```python
from build123d import *

# Parameters (mm, degrees)
SKETCH_1_W          = 27.8
SKETCH_1_H          = 8
EXTRUDE_1_DEPTH     = 7.8
EXTRUDE_2_DEPTH     = 27.8
SKETCH_4_R          = 1.15
EXTRUDE_3_DEPTH     = 2
CUT_EXTRUDE_4_DEPTH = 24.8
SKETCH_15_W         = 27.8
SKETCH_15_H         = 4.251772847
EXTRUDE_4_DEPTH     = 1.9
FILLET_1_R          = 8
FILLET_2_R          = 6.5
EXTRUDE_5_DEPTH     = 27.8
CUT_EXTRUDE_6_DEPTH = 24.8
SKETCH_19_OUTSIDE_W = 26.556
SKETCH_19_OUTSIDE_H = 34.032
CUT_EXTRUDE_7_DEPTH = 40.8
SKETCH_20_W         = 1.5
SKETCH_20_H         = 5.56
EXTRUDE_6_DEPTH     = 6.2
SKETCH_21_W         = 1.5
SKETCH_21_H         = 3.16
CUT_EXTRUDE_8_DEPTH = 4.68
EXTRUDE_7_DEPTH     = 1
FILLET_3_R          = 0.2


with BuildPart() as part:
    # 草图1 → 凸台-拉伸1 (new body)
    with BuildSketch(Plane.XY):
        with Locations((13.9, -4)):
            Rectangle(SKETCH_1_W, SKETCH_1_H)
    extrude(amount=EXTRUDE_1_DEPTH)

    # 草图2 → 凸台-拉伸2 (add)
    with BuildSketch(Plane.ZY):
        Polygon((5.795554958, -15.947085729), (0, -17.5), (0, -8), (7.8, -8), align=None)
    extrude(amount=-EXTRUDE_2_DEPTH)

    # 草图4 → 凸台-拉伸3 (add)
    with BuildSketch(Plane(origin=(0, 0, -1.9), x_dir=(-1, 0, 0), z_dir=(0, 0, -1))):
        with BuildLine():
            Line((0, -2), (0, -4.7))
            Line((0, -4.7), (6, -4.7))
            ThreePointArc((6, -4.7), (6.353553391, -4.553553391), (6.5, -4.2))
            Line((6.5, -4.2), (6.5, -2))
            Line((6.5, -2), (6.5, 2.4))
            ThreePointArc((6.5, 2.4), (6.353553391, 2.753553391), (6, 2.9))
            Line((6, 2.9), (4, 2.9))
            ThreePointArc((4, 2.9), (2.232233047, 2.167766953), (1.5, 0.4))
            Line((1.5, 0.4), (1.5, -1.8))
            ThreePointArc((1.5, -1.8), (1.441421356, -1.941421356), (1.3, -2))
            Line((1.3, -2), (0, -2))
        make_face()
        with Locations((3.6, 0.5)):
            Circle(SKETCH_4_R, mode=Mode.SUBTRACT)
    extrude_3 = extrude(amount=-EXTRUDE_3_DEPTH)

    # 镜向1: 凸台-拉伸3 across plane
    add(extrude_3.mirror(Plane.ZY.offset(-13.9)))

    # 草图13 → 切除-拉伸4 (cut)
    with BuildSketch(Plane.ZY.offset(-1.5)):
        Polygon((1.5, 0), (1.5, -11.921695309), (0, -12.323619098), (0, -15.947085729), (4.556522218, -14.726169281), (6.3, -7.813748582), (6.3, 0), align=None)
    extrude(amount=-CUT_EXTRUDE_4_DEPTH, mode=Mode.SUBTRACT)

    # 草图15 → 凸台-拉伸4 (add)
    with BuildSketch(Plane(origin=(0, 0, 0), x_dir=(-1, 0, 0), z_dir=(0, 0, -1))):
        with Locations((-13.9, -4.125886424)):
            Rectangle(SKETCH_15_W, SKETCH_15_H)
    extrude(amount=EXTRUDE_4_DEPTH)

    # 圆角1
    fillet_1_edges = [part.edges().sort_by_distance(p)[0] for p in [
        (13.9, -14.726169281, 4.556522218),
    ]]
    fillet(fillet_1_edges, radius=FILLET_1_R)

    # 圆角2
    fillet_2_edges = [part.edges().sort_by_distance(p)[0] for p in [
        (13.9, -15.947085729, 5.795554958),
    ]]
    fillet(fillet_2_edges, radius=FILLET_2_R)

    # 草图17 → 凸台-拉伸5 (add)
    with BuildSketch(Plane(origin=(27.8, 0, 0), x_dir=(0, 0, -1), z_dir=(1, 0, 0))):
        Polygon((0, -17.5), (7, -19.375644347), (7, -12.646349174), (0, -10.770704827), align=None)
    extrude(amount=-EXTRUDE_5_DEPTH)

    # 草图18 → 切除-拉伸6 (cut)
    with BuildSketch(Plane.ZY.offset(-26.3)):
        Polygon((0, -12.323619098), (0, -15.947085729), (-7, -17.822730076), (-7, -14.199263445), align=None)
    extrude(amount=CUT_EXTRUDE_6_DEPTH, mode=Mode.SUBTRACT)

    # 草图19 outside → 切除-拉伸7 (cut)
    with BuildSketch(Plane(origin=(34.3, 0, 0), x_dir=(0, 0, -1), z_dir=(1, 0, 0))):
        with Locations((-0.4, -8.238)):
            Rectangle(SKETCH_19_OUTSIDE_W, SKETCH_19_OUTSIDE_H)
        Polygon((7, 2.9), (7, -14.199263445), (-1.5, -11.921695309), (-1.5, 2.9), align=None, mode=Mode.SUBTRACT)
    extrude(amount=-CUT_EXTRUDE_7_DEPTH, mode=Mode.SUBTRACT)

    # 草图20 → 凸台-拉伸6 (add)
    with BuildSketch(Plane(origin=(0, -7.983041289, 0), x_dir=(1, 0, 0), z_dir=(0, 0, -1))):
        with Locations((-0.75, 0.007663538)):
            Rectangle(SKETCH_20_W, SKETCH_20_H)
    extrude_6 = extrude(amount=-EXTRUDE_6_DEPTH)

    # 草图21 → 切除-拉伸8 (cut)
    with BuildSketch(Plane(origin=(0, -7.983041289, 0), x_dir=(1, 0, 0), z_dir=(0, 0, -1))):
        with Locations((-0.75, 0.007663538)):
            Rectangle(SKETCH_21_W, SKETCH_21_H)
    cut_extrude_8 = extrude(amount=-CUT_EXTRUDE_8_DEPTH, mode=Mode.SUBTRACT)

    # 镜向2: 凸台-拉伸6, 切除-拉伸8 across plane
    add(extrude_6.mirror(Plane.ZY.offset(-13.9)))
    add(cut_extrude_8.mirror(Plane.ZY.offset(-13.9)), mode=Mode.SUBTRACT)

    # 草图23 → 凸台-拉伸7 (add)
    with BuildSketch(Plane.ZY.offset(-1)):
        Polygon((1.5, 0), (1.5, -11.921695309), (-7, -14.199263445), (-7, -14.923956771), (2.2, -12.458824201), (2.2, 0), align=None)
    extrude_7 = extrude(amount=-EXTRUDE_7_DEPTH)

    # 镜向3: 凸台-拉伸7 across plane
    add(extrude_7.mirror(Plane.ZY.offset(-13.9)))

    # 圆角3
    fillet_3_edges = [part.edges().sort_by_distance(p)[0] for p in [
        (-0.75, -5.210704827, 6.2),
        (-0.75, -10.770704827, 6.2),
        (28.55, -10.770704827, 6.2),
        (28.55, -5.210704827, 6.2),
    ]]
    fillet(fillet_3_edges, radius=FILLET_3_R)


solid = part.part
```
Could you check a few things on this model? Use its own coordinates, in mm. A direction names the side the tool comes from. Give positions to 0.01 mm unless a question says otherwise; leave off trailing zeros. Write each loop counter-clockwise with the first axis right and the second up, starting at its lowest first coordinate (ties: lowest second). Pieces come first, ordered by that corner, then holes. Notation, with made-up numbers: (30, 16.25) - (59, 16.25) arc R22 cw to (59, 51.25) - close; hole circle Ø8 at (52, -9.5). An arc over 180 degrees is marked (long way). One line per item, written item: value. Start each with the question number.
Item 1: Please list where these lines run through material, in increasing order: line 1 (Z direction, x = 18.5, y = -0.5); line 2 (Y direction, x = -3.6, z = -1.1); line 3 (Z direction, x = 26, y = -7). Write a range as from..to.
Item 2: Imagine slicing it at A-A, the plane z = 4.25. List the corners of the cut face in (x, y) for me.
Item 3: Imagine slicing it at C-C, the plane x = 31. List the corners of the cut face in (y, z) for me.
Item 4: Imagine slicing it at B-B, the plane z = -1. Give the number of separate pieces and of enclosed holes in the cut face, and give its area (3 significant figures).
Item 5: If we mould it in two halves opening along X, with no side actions, what happens to faces 5 (the face through (29.3, -8, 5)), 6 (the face through (14, -2, -1)), 7 (the face through (29, -10.771, 3))? For each: +X half, -X half, draft (parallel to the pull), parting line (faces both ways), or undercut.
Item 6: I'm going to push flat-ended pins straight in: pin 1 (1.5 mm diameter, centred on x = 14, y = -8.5, fed in from -Z); pin 2 (2 mm diameter, centred on x = -4, z = -0.5, fed in from -Y); pin 3 (7 mm diameter, centred on x = 32, y = -0.5, fed in from +Z). Where does each tip first touch, or does it pass through?
Item 7: Imagine slicing it at D-D, the plane x = 10. List the corners of the cut face in (y, z) for me.
Item 8: Which directions (+Z, -Z, +X, -X, +Y, -Y) give clear straight access to the entire face, cutting with the end or side of a thin tool? Please do faces 1 (the face through (0, -8, 5)), 2 (the face through (26.8, -9, 2)), 3 (the face through (29.3, -1, -1)), 4 (the face through (-1, -6.411, 2)).
Geometry says:
1. line 1: 0..1.5
1. line 2: -4.7..-0.65, 1.65..2.87
1. line 3: 0..2.2
2. outline: (-1.5, -10.77) - (0, -10.77) - (0, -9.57) - (-1.5, -9.57) - close; (-1.5, -6.41) - (0, -6.41) - (0, -5.21) - (-1.5, -5.21) - close; (27.8, -10.77) - (29.3, -10.77) - (29.3, -9.57) - (27.8, -9.57) - close; (27.8, -6.41) - (29.3, -6.41) - (29.3, -5.21) - (27.8, -5.21) - close
3. outline: (-4.7, -1.9) - (-0.58, -1.9) - (-0.58, 0.1) - (-4.7, 0.1) - close; (1.58, -1.9) - (2.77, -1.9) - (2.77, 0.1) - (1.58, 0.1) - close
4. separate pieces: 2
4. enclosed holes: 2
4. area: 236 mm^2
5. face 5: +X half
5. face 6: undercut
5. face 7: draft
6. pin 1: z = 0
6. pin 2: y = -4.7
6. pin 3: z = 0.1
7. outline: (-14.2, -7) - (-12.65, -7) - (-10.77, 0) - (-6.25, 0) - (-6.25, -1.9) - (-2, -1.9) - (-2, 0) - (0, 0) - (0, 1.5) - (-11.92, 1.5) - close
8. face 1: +Z, +Y, -Y
8. face 2: +Z, -Y
8. face 3: +Z, -Z, +Y
8. face 4: -Z, -X
